Here's how the part is built. I have some questions about the finished solid (model axes, mm). Round coordinates to 2 decimals unless told otherwise and drop trailing zeros. Loops run counter-clockwise (first coordinate to the right, second up) from the corner with the lowest first, then second, coordinate; pieces in that order, holes last. Notation, with made-up numbers: M 6.5,84 L 29.5,84 A14 ccw 29.5,111 Z; hole C 68.5,31.25 d4. An arc over 180 degrees is marked long. Use a Markdown table: item, result.
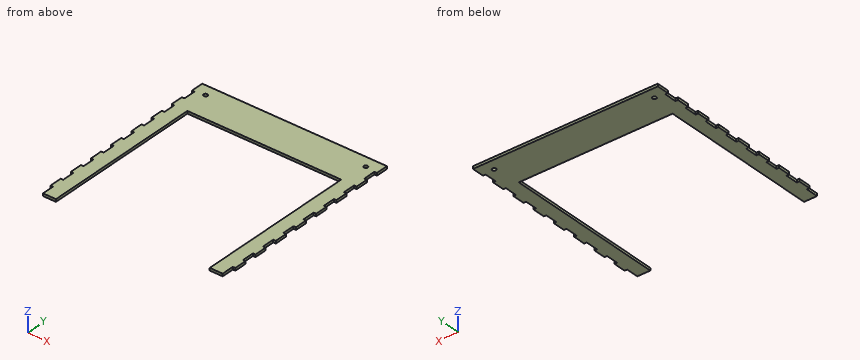
```python
from build123d import *

# Parameters (mm, degrees)
SKETCH1_R           = 4
BOSS_EXTRUDE1_DEPTH = 5.207


with BuildPart() as part:
    # Sketch1 → Boss-Extrude1 (new body)
    with BuildSketch(Plane.XY):
        Polygon((-184.15, 25.4), (-184.15, 0), (-157.607, 0), (-157.607, 330.2), (157.607, 330.2), (157.607, 0), (184.15, 0), (184.15, 25.4), (189.357, 25.4), (189.357, 50.8), (184.15, 50.8), (184.15, 76.2), (189.357, 76.2), (189.357, 101.6), (184.15, 101.6), (184.15, 127), (189.357, 127), (189.357, 152.4), (184.15, 152.4), (184.15, 177.8), (189.357, 177.8), (189.357, 203.2), (184.15, 203.2), (184.15, 228.6), (189.357, 228.6), (189.357, 254), (184.15, 254), (184.15, 279.4), (189.357, 279.4), (189.357, 304.8), (184.15, 304.8), (184.15, 330.2), (189.357, 330.2), (189.357, 355.6), (184.15, 355.6), (184.15, 381), (189.357, 381), (189.357, 406.4), (-189.357, 406.4), (-189.357, 381), (-184.15, 381), (-184.15, 355.6), (-189.357, 355.6), (-189.357, 330.2), (-184.15, 330.2), (-184.15, 304.8), (-189.357, 304.8), (-189.357, 279.4), (-184.15, 279.4), (-184.15, 254), (-189.357, 254), (-189.357, 228.6), (-184.15, 228.6), (-184.15, 203.2), (-189.357, 203.2), (-189.357, 177.8), (-184.15, 177.8), (-184.15, 152.4), (-189.357, 152.4), (-189.357, 127), (-184.15, 127), (-184.15, 101.6), (-189.357, 101.6), (-189.357, 76.2), (-184.15, 76.2), (-184.15, 50.8), (-189.357, 50.8), (-189.357, 25.4), align=None)
        with Locations((-164.150000122, 384.05)):
            Circle(SKETCH1_R, mode=Mode.SUBTRACT)
        with Locations((164.1499892, 384.05)):
            Circle(SKETCH1_R, mode=Mode.SUBTRACT)
    extrude(amount=BOSS_EXTRUDE1_DEPTH)


solid = part.part
```
Q1. I need wall thicknesses on line 1 (X direction, y = 384.05, z = 2.2); line 2 (X direction, y = 70.5, z = 1.4); line 3 (X direction, y = 97, z = 4.8). Which ranges of each line are inside material? Lowest first, please. Write a range as from..to.
Return value:
| item | result |
|---|---|
| line 1 | x = -189.36..-168.15, -160.15..160.15, 168.15..189.36 |
| line 2 | x = -184.15..-157.61, 157.61..184.15 |
| line 3 | x = -189.36..-157.61, 157.61..189.36 |
Q2. Imagine slicing it at C-C, the plane x = -87.5. Please give me the cut outline in (y, z).
Return value:
| item | result |
|---|---|
| outline | M 330.2,0 L 406.4,0 L 406.4,5.21 L 330.2,5.21 Z |
Q3. Will these pins go through, and if not, where does the flat tip stop? P1, Ø2.5, axis at y = 11, z = 2.5, coming from the -X side; P2, Ø1.6, axis at y = 370, z = 2.5, coming from the +X side; P3, Ø1.6, axis at x = -186.5, z = 2, coming from the -Y side.
Return value:
| item | result |
|---|---|
| P1 | stops at x = -184.15 |
| P2 | stops at x = 184.15 |
| P3 | stops at y = 25.4 |
Q4. Imagine slicing it at B-B, the plane z = 2.6. Give the number of separate pieces and of enclosed holes in the cut face, then the cut area to 3 significant figures.
Return value:
| item | result |
|---|---|
| separate pieces | 1 |
| enclosed holes | 2 |
| area | 47,600 mm^2 |
Q5. Imagine slicing it at A-A, the plane y = 310.5. Please give me the cut outline in (x, z).
Return value:
| item | result |
|---|---|
| outline | M -184.15,0 L -157.61,0 L -157.61,5.21 L -184.15,5.21 Z; M 157.61,0 L 184.15,0 L 184.15,5.21 L 157.61,5.21 Z |
